Here's how the part is built. I have some questions about the finished solid (model axes, mm). A direction names the side the tool comes from. Give positions to 0.01 mm unless a question says otherwise; leave off trailing zeros. Loops run counter-clockwise (first coordinate to the right, second up) from the corner with the lowest first, then second, coordinate; pieces in that order, holes last.
Q1. If we section it at B-B (x = 5): Please give me the cut outline in (y, z).
Q2. We'd pull the mould along Y, two halves only. Please class faces 4 (the face through (0, 0, -3)), 5 (the face through (6.6, 25.1, 0.8)), 6 (the face through (7.5, 15, -1)): +Y half, -Y half, draft (parallel to the pull), parting line (faces both ways), or undercut.
Q3. For faces 1 (the face through (-6.6, 25.1, 0.8)), 2 (the face through (-7, 15, 0.275)), 3 (the face through (6.5, 28, 1)), which set-ups out of +Z, -Z, +X, -X, +Y, -Y let a thin tool reach every point of the face, with its end or its side?
Q4. Will these pins go through, and if not, where does the flat tip stop? P1, Ø1.9, axis at x = 5, y = 25.1, coming from the -Z side; P2, Ø12, axis at x = -1, y = 8.5, coming from the +Z side.
Q5. If we section it at D-D (y = 21.5): Please give me the cut outline in (x, z), plus the area to 3 significant figures.
Q6. If we section it at A-A (y = 25.1): Please give me the cut outline in (x, z), plus the area to 3 significant figures.
Q7. I need wall thicknesses on line 1 (Y direction, x = 5, z = -3.25); line 2 (X direction, y = 14, z = -0.5); line 3 (Z direction, x = 6, y = 13). Which ranges of each line are inside material? Lowest first, please.
Q8. If we section it at C-C (z = -3): Please give me the cut outline in (x, y), plus the area to 3 significant figures.
from build123d import *

# Parameters (mm, degrees)
EXTRUDE_1_DEPTH     = 31.2
SKETCH_2_R          = 1.6
CUT_EXTRUDE_1_DEPTH = 10


with BuildPart() as part:
    # 草图1 → 凸台-拉伸1 (new body)
    with BuildSketch(Plane(origin=(0, 0, 0), x_dir=(1, 0, 0), z_dir=(0, 1, 0))):
        Polygon((-7.5, -0.275116875), (-6.5, -0.275116875), (-6.5, -1.275116875), (-15.6, -1.275116875), (-15.6, 5.824883125), (15.6, 5.824883125), (15.6, -1.275116875), (6.5, -1.275116875), (6.5, -0.275116875), (7.5, -0.275116875), (7.5, 2.224883125), (-7.5, 2.224883125), align=None)
    extrude(amount=EXTRUDE_1_DEPTH)

    # 草图2 → 切除-拉伸1 (cut)
    with BuildSketch(Plane(origin=(0, 0, -5.824883125), x_dir=(-1, 0, 0), z_dir=(0, 0, -1))):
        with Locations((-5, 25.1)):
            Circle(SKETCH_2_R)
        with Locations((5, 25.1)):
            Circle(SKETCH_2_R)
        with Locations((5, 6.1)):
            Circle(SKETCH_2_R)
        with Locations((-5, 6.1)):
            Circle(SKETCH_2_R)
    extrude(amount=-CUT_EXTRUDE_1_DEPTH, mode=Mode.SUBTRACT)


solid = part.part
Check sheet entries:
1. outline: (0, -5.82) - (4.5, -5.82) - (4.5, -2.22) - (0, -2.22) - close; (7.7, -5.82) - (23.5, -5.82) - (23.5, -2.22) - (7.7, -2.22) - close; (26.7, -5.82) - (31.2, -5.82) - (31.2, -2.22) - (26.7, -2.22) - close
2. face 4: -Y half
2. face 5: undercut
2. face 6: draft
3. face 1: +Z, -Z
3. face 2: +Y, -Y
3. face 3: +Z, +Y, -Y
4. P1: passes through
4. P2: stops at z = 1.28
5. outline: (-15.6, -5.82) - (15.6, -5.82) - (15.6, 1.28) - (6.5, 1.28) - (6.5, 0.28) - (7.5, 0.28) - (7.5, -2.22) - (-7.5, -2.22) - (-7.5, 0.28) - (-6.5, 0.28) - (-6.5, 1.28) - (-15.6, 1.28) - close
5. area: 171 mm2
6. outline: (-15.6, -5.82) - (-6.6, -5.82) - (-6.6, -2.22) - (-7.5, -2.22) - (-7.5, 0.28) - (-6.6, 0.28) - (-6.6, 1.28) - (-15.6, 1.28) - close; (-3.4, -5.82) - (3.4, -5.82) - (3.4, -2.22) - (-3.4, -2.22) - close; (6.6, -5.82) - (15.6, -5.82) - (15.6, 1.28) - (6.6, 1.28) - (6.6, 0.28) - (7.5, 0.28) - (7.5, -2.22) - (6.6, -2.22) - close
6. area: 148 mm2
7. line 1: y = 0 to 4.5, 7.7 to 23.5, 26.7 to 31.2
7. line 2: x = -15.6 to -7.5, 7.5 to 15.6
7. line 3: z = -5.82 to -2.22
8. outline: (-15.6, 0) - (15.6, 0) - (15.6, 31.2) - (-15.6, 31.2) - close; hole circle Ø3.2 at (-5, 6.1); hole circle Ø3.2 at (-5, 25.1); hole circle Ø3.2 at (5, 6.1); hole circle Ø3.2 at (5, 25.1)
8. area: 941 mm2
